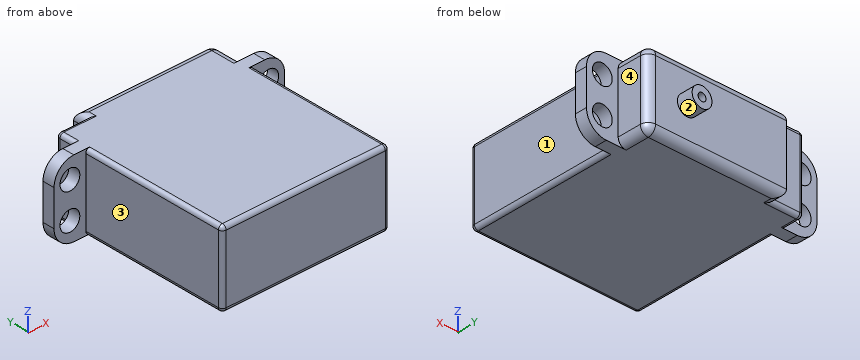
```python
from build123d import *

# Parameters (mm, degrees)
SKETCH1_W           = 42.162271806
SKETCH1_H           = 37
SKETCH1_W_2         = 35
SKETCH1_H_2         = 3
BOSS_EXTRUDE1_DEPTH = 19
SKETCH2_R           = 2.5
CUT_EXTRUDE1_DEPTH  = 19
SKETCH4_R           = 2.5
SKETCH4_R_2         = 1
BOSS_EXTRUDE2_DEPTH = 4
FILLET1_R           = 2
FILLET2_R           = 2
FILLET3_R           = 5
FILLET4_R           = 1
FILLET5_R           = 1


with BuildPart() as part:
    # Sketch1 → Boss-Extrude1 (new body)
    with BuildSketch(Plane.XY):
        with Locations((3.738336714, 20.81643002)):
            Rectangle(SKETCH1_W, SKETCH1_H)
        Polygon((-25.342799189, 39.31643002), (-17.342799189, 39.31643002), (24.819472617, 39.31643002), (32.819472617, 39.31643002), (32.819472617, 42.31643002), (24.819472617, 42.31643002), (-17.342799189, 42.31643002), (-25.342799189, 42.31643002), align=None)
        Polygon((-17.342799189, 47.31643002), (-17.342799189, 42.31643002), (24.819472617, 42.31643002), (24.819472617, 47.31643002), (-10.180527383, 47.31643002), align=None)
        with Locations((7.319472617, 48.81643002)):
            Rectangle(SKETCH1_W_2, SKETCH1_H_2)
    extrude(amount=BOSS_EXTRUDE1_DEPTH)

    # Sketch2 → Cut-Extrude1 (cut)
    with BuildSketch(Plane(origin=(0, 42.31643002, 0), x_dir=(1, 0, 0), z_dir=(0, 1, 0))):
        with Locations(Location((-21.342799189, -14, 0), (0, 0, 270))):
            Circle(SKETCH2_R)
        with Locations(Location((-21.342799189, -5, 0), (0, 0, 270))):
            Circle(SKETCH2_R)
        with Locations(Location((28.819472617, -5, 0), (0, 0, 270))):
            Circle(SKETCH2_R)
        with Locations(Location((28.819472617, -14, 0), (0, 0, 270))):
            Circle(SKETCH2_R)
    extrude(amount=-CUT_EXTRUDE1_DEPTH, mode=Mode.SUBTRACT)

    # Sketch4 → Boss-Extrude2 (add)
    with BuildSketch(Plane(origin=(0, 50.31643002, 0), x_dir=(1, 0, 0), z_dir=(0, 1, 0))):
        with Locations(Location((14.819472617, -9.5, 0), (0, 0, 270))):
            Circle(SKETCH4_R)
        with Locations(Location((14.819472617, -9.5, 0), (0, 0, 270))):
            Circle(SKETCH4_R_2, mode=Mode.SUBTRACT)
    extrude(amount=BOSS_EXTRUDE2_DEPTH)

    # Fillet1
    fillet1_edges = [part.edges().sort_by_distance(p)[0] for p in [
        (-10.180527383, 48.81643002, 0),
        (-10.180527383, 48.81643002, 19),
    ]]
    fillet(fillet1_edges, radius=FILLET1_R)

    # Fillet2
    # the kernel refuses this fillet: 2 mm, written as the material it takes off along each edge
    with BuildSketch(Plane(origin=(22.819472617, 48.31643002, 2), x_dir=(1, 0, 0), z_dir=(0, 0, -1))) as fillet2_piece_1_section:
        Polygon((0, 0), (FILLET2_R * 1.02, 0), (FILLET2_R * 1.02, -FILLET2_R * 1.02), (0, -FILLET2_R * 1.02), align=None)
    fillet2_piece_1 = extrude(amount=FILLET2_R * 1.02, mode=Mode.PRIVATE)
    fillet2_piece_1 = fillet2_piece_1 - Plane(origin=(22.819472617, 48.31643002, 2), x_dir=(-0.7071067811865475, -0.7071067811865475, 0), z_dir=(0, 0, -1)) * Sphere(FILLET2_R, mode=Mode.PRIVATE)
    add(fillet2_piece_1, mode=Mode.SUBTRACT)
    with BuildSketch(Plane(origin=(22.819472617, 48.31643002, 17), x_dir=(0, 0, 1), z_dir=(1, 0, 0))) as fillet2_piece_2_section:
        Polygon((0, 0), (FILLET2_R * 1.02, 0), (FILLET2_R * 1.02, -FILLET2_R * 1.02), (0, -FILLET2_R * 1.02), align=None)
    fillet2_piece_2 = extrude(amount=FILLET2_R * 1.02, mode=Mode.PRIVATE)
    fillet2_piece_2 = fillet2_piece_2 - Plane(origin=(22.819472617, 48.31643002, 17), x_dir=(0, -0.7071067811865475, -0.7071067811865475), z_dir=(1, 0, 0)) * Sphere(FILLET2_R, mode=Mode.PRIVATE)
    add(fillet2_piece_2, mode=Mode.SUBTRACT)
    with BuildSketch(Plane(origin=(22.819472617, 50.31643002, 0), x_dir=(0, -1, 0), z_dir=(-1, 0, 0))) as fillet2_piece_3:
        with BuildLine():
            CenterArc((FILLET2_R, FILLET2_R), FILLET2_R, 180, 90)
            Line((0, FILLET2_R), (0, 0))
            Line((0, 0), (FILLET2_R, 0))
        make_face()
    extrude(amount=36, mode=Mode.SUBTRACT)
    with BuildSketch(Plane(origin=(24.819472617, 48.31643002, 0), x_dir=(-1, 0, 0), z_dir=(0, -1, 0))) as fillet2_piece_4:
        with BuildLine():
            CenterArc((FILLET2_R, -FILLET2_R), FILLET2_R, 90, 90)
            Line((0, -FILLET2_R), (0, 0))
            Line((0, 0), (FILLET2_R, 0))
        make_face()
    extrude(amount=6, mode=Mode.SUBTRACT)
    with BuildSketch(Plane(origin=(24.819472617, 42.31643002, 19), x_dir=(0, 0, -1), z_dir=(0, 1, 0))) as fillet2_piece_5:
        with BuildLine():
            CenterArc((FILLET2_R, FILLET2_R), FILLET2_R, 180, 90)
            Line((0, FILLET2_R), (0, 0))
            Line((0, 0), (FILLET2_R, 0))
        make_face()
    extrude(amount=6, mode=Mode.SUBTRACT)
    with BuildSketch(Plane(origin=(22.819472617, 50.31643002, 19), x_dir=(0, -1, 0), z_dir=(-1, 0, 0))) as fillet2_piece_6:
        with BuildLine():
            CenterArc((FILLET2_R, -FILLET2_R), FILLET2_R, 90, 90)
            Line((0, -FILLET2_R), (0, 0))
            Line((0, 0), (FILLET2_R, 0))
        make_face()
    extrude(amount=36, mode=Mode.SUBTRACT)
    with BuildSketch(Plane(origin=(24.819472617, 50.31643002, 2), x_dir=(0, -1, 0), z_dir=(0, 0, 1))) as fillet2_piece_7:
        with BuildLine():
            CenterArc((FILLET2_R, -FILLET2_R), FILLET2_R, 90, 90)
            Line((0, -FILLET2_R), (0, 0))
            Line((0, 0), (FILLET2_R, 0))
        make_face()
    extrude(amount=15, mode=Mode.SUBTRACT)

    # Fillet3
    fillet3_edges = [part.edges().sort_by_distance(p)[0] for p in [
        (-25.342799189, 40.81643002, 0),
        (32.819472617, 40.81643002, 19),
        (32.819472617, 40.81643002, 0),
        (-25.342799189, 40.81643002, 19),
    ]]
    fillet(fillet3_edges, radius=FILLET3_R)

    # Fillet4
    fillet4_edges = [part.edges().sort_by_distance(p)[0] for p in [
        (-17.342799189, 44.81643002, 0),
        (-12.761663286, 47.31643002, 0),
        (-17.342799189, 47.31643002, 9.5),
        (-12.761663286, 47.31643002, 19),
        (-17.342799189, 44.81643002, 19),
    ]]
    fillet(fillet4_edges, radius=FILLET4_R)

    # Fillet5
    fillet5_edges = [part.edges().sort_by_distance(p)[0] for p in [
        (24.819472617, 20.81643002, 19),
        (-17.342799189, 20.81643002, 0),
        (24.819472617, 20.81643002, 0),
        (3.738336714, 2.31643002, 0),
        (-17.342799189, 2.31643002, 9.5),
        (24.819472617, 2.31643002, 9.5),
        (3.738336714, 2.31643002, 19),
        (-17.342799189, 20.81643002, 19),
    ]]
    fillet(fillet5_edges, radius=FILLET5_R)


solid = part.part
```
Verification items for the finished model (mm, model axes). Face numbers are marked on the shaded views. A direction names the side the tool comes from. Coordinates: 2 decimals unless noted, no trailing zeros. Write each loop counter-clockwise with the first axis right and the second up, starting at its lowest first coordinate (ties: lowest second). Pieces come first, ordered by that corner, then holes. Notation, with made-up numbers: M 81.5,-2.75 L 135.5,-2.75 A22 ccw 135.5,20.25 Z; hole C 12.25,-3 d3. An arc over 180 degrees is marked long. Answer as a JSON object with one key per item and string values. Group by question number.
(1) Cross-section at B-B, the plane y = 27. Record the cut outline in (x, z).
(2) Gauge pin test, flat ends, axial feed: pin 1 (6.5 mm diameter, centred on x = 28.82, z = 5, fed in from -Y); pin 2 (3 mm diameter, centred on y = 18, z = 8.5, fed in from -X); pin 3 (2 mm diameter, centred on x = -13, z = 14, fed in from +Y); pin 4 (3 mm diameter, centred on x = 28.82, z = 14, fed in from -Y). Record the tip position at first contact, or that the pin passes through.
(3) Tool access check on the marked faces 1, 2, 3 and 4. Record the directions out of +Z, -Z, +X, -X, +Y, -Y that give a thin tool (end or side, any length) a straight path to the whole face; none if there is none.
(4) Cross-section at A-A, the plane z = 9.5. Record the cut outline in (x, y).
(5) Material ranges on line 1 (X direction, y = 39.95, z = 5); line 2 (Z direction, x = -21, y = 41); line 3 (X direction, y = 52.25, z = 9.5), recorded low to high.
(6) Cross-section at C-C, the plane x = 5. Record the cut outline in (y, z).
Reply:
{
 "1": {"outline": "M -17.34,1 A1 ccw -16.34,0 L 23.82,0 A1 ccw 24.82,1 L 24.82,18 A1 ccw 23.82,19 L -16.34,19 A1 ccw -17.34,18 Z"},
 "2": {"pin 1": "y = 39.32", "pin 2": "x = -17.34", "pin 3": "y = 47.32", "pin 4": "through"},
 "3": {"face 1": "+Z, -Z, +X, -Y", "face 2": "+Y", "face 3": "+Z, -Z, -X, -Y", "face 4": "+Z, -Z, +X, +Y"},
 "4": {"outline": "M -25.34,39.32 L -17.34,39.32 L -17.34,3.32 A1 ccw -16.34,2.32 L 23.82,2.32 A1 ccw 24.82,3.32 L 24.82,39.32 L 32.82,39.32 L 32.82,42.32 L 24.82,42.32 L 24.82,48.32 A2 ccw 22.82,50.32 L 17.32,50.32 L 17.32,54.32 L 15.82,54.32 L 15.82,50.32 L 13.82,50.32 L 13.82,54.32 L 12.32,54.32 L 12.32,50.32 L -10.18,50.32 L -10.18,47.32 L -16.34,47.32 A1 ccw -17.34,46.32 L -17.34,42.32 L -25.34,42.32 Z"},
 "5": {"line 1": "-25.34 to -23.84, -18.84 to 26.32, 31.32 to 32.82", "line 2": "0.04 to 2.52, 7.48 to 11.52, 16.48 to 18.96", "line 3": "12.32 to 13.82, 15.82 to 17.32"},
 "6": {"outline": "M 2.32,1 A1 ccw 3.32,0 L 48.32,0 A2 ccw 50.32,2 L 50.32,17 A2 ccw 48.32,19 L 3.32,19 A1 ccw 2.32,18 Z"}
}
